```python
from build123d import *

# Parameters (mm, degrees)
F0_W           = 65
F0_H           = 38
F1_DEPTH       = 2
F2_W           = 34
F2_H           = 4
F3_DEPTH       = 48.95
F5_R           = 3.5
F6_DEPTH       = 3000
F4_R           = 25
F7_DEPTH       = 12
F9_R           = 3
F10_DEPTH      = 38
F11_R          = 25
F12_DEPTH      = 12
F12_DEPTH_BACK = 12


with BuildPart() as f1:
    # F0 (on Top) → F1 (new body)
    with BuildSketch(Plane.XY):
        Rectangle(F0_W, F0_H)
    extrude(amount=F1_DEPTH)

    # F2 (on face) → F3 (join)
    with BuildSketch(Plane(origin=(0, 0, 0), x_dir=(1, 0, 0), z_dir=(0, 0, -1))):
        with Locations((0, 17)):
            Rectangle(F2_W, F2_H)
        with Locations((0, -17)):
            Rectangle(F2_W, F2_H)
    extrude(amount=F3_DEPTH)

    # F5 (on face) → F6 (cut)
    with BuildSketch(Plane.XY.offset(2)):
        with Locations((27, 12)):
            Circle(F5_R)
        with Locations((27, -12)):
            Circle(F5_R)
        with Locations((-27, -12)):
            Circle(F5_R)
        with Locations((-27, 12)):
            Circle(F5_R)
    extrude(amount=-F6_DEPTH, mode=Mode.SUBTRACT)

    # F9 (on face) → F10 (join)
    with BuildSketch(Plane(origin=(0, 19, 0), x_dir=(-1, 0, 0), z_dir=(0, 1, 0))):
        with Locations((0, -43)):
            Circle(F9_R)
    extrude(amount=-F10_DEPTH)

    # F11 (on Front) → F12 (join, two sides)
    with BuildSketch(Plane.XZ) as f12_sk:
        with Locations((0, -43)):
            Circle(F11_R)
    extrude(amount=F12_DEPTH)
    extrude(f12_sk.sketch, amount=-F12_DEPTH_BACK)


with BuildPart() as f7:
    # F4 (on Front) → F7 (new body, symmetric)
    with BuildSketch(Plane.XZ):
        with Locations((0, -43)):
            Circle(F4_R)
    extrude(amount=F7_DEPTH, both=True)


solid = f1.part
```
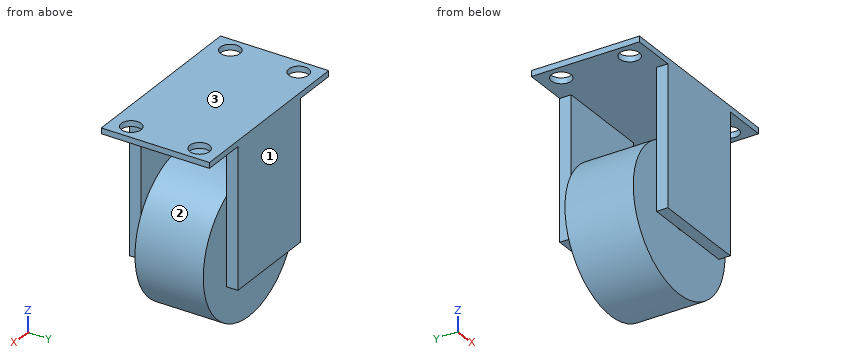
Can you work these out from the model? Positions are in its coordinate system, mm. Face numbers are marked on the shaded views. Round coordinates to 2 decimals unless told otherwise and drop trailing zeros. Loops run counter-clockwise (first coordinate to the right, second up) from the corner with the lowest first, then second, coordinate; pieces in that order, holes last. Notation, with made-up numbers: M 9.5,-29.75 L 51.5,-29.75 A19 ccw 51.5,4.25 Z; hole C 12.25,53 d4. An arc over 180 degrees is marked long. Answer as a JSON object with one key per item and string values. Group by question number.
Q1. Imagine slicing it at D-D, the plane z = -24.5. Please give me the cut outline in (x, y).
Q2. Imagine slicing it at B-B, the plane y = -1. Please give me the cut outline in (x, z), then the cut area to 3 significant figures.
Q3. Will these pins go through, and if not, where does the flat tip stop? pin 1 (3 mm diameter, centred on y = 7, z = -20, fed in from +X); pin 2 (10 mm diameter, centred on y = -8.5, z = -18, fed in from -X); pin 3 (10 mm diameter, centred on y = -2, z = -23.5, fed in from -X).
Q4. Imagine slicing it at A-A, the plane x = 27. Please give me the cut outline in (y, z), then the cut area to 3 significant figures.
Q5. Please list where these lines run through material, in increasing order: L1, parallel to Y at x = -27, z = 0.45; L2, parallel to Y at x = 16.5, z = -29; L3, parallel to Z at x = -4, y = -14.
Q6. We'd pull the mould along Z, two halves only. Please class the marked faces 1, 2 and 3: +Z half, -Z half, draft (parallel to the pull), parting line (faces both ways), or undercut.
Q7. Imagine slicing it at C-C, the plane x = 18. Please give me the cut outline in (y, z).
Findings:
{
 "1": {"outline": "M -17,-19 L 17,-19 L 17,-15 L -17,-15 Z; M -17,15 L 17,15 L 17,19 L -17,19 Z; M -16.82,-12 L 16.82,-12 L 16.82,12 L -16.82,12 Z"},
 "2": {"outline": "M -32.5,0 L 32.5,0 L 32.5,2 L -32.5,2 Z; C 0,-43 d50", "area": "2,090 mm2"},
 "3": {"pin 1": "stops at x = 12.76", "pin 2": "stops at x = -15", "pin 3": "stops at x = -20.37"},
 "4": {"outline": "M -19,0 L -15.5,0 L -15.5,2 L -19,2 Z; M -8.5,0 L 8.5,0 L 8.5,2 L -8.5,2 Z; M 15.5,0 L 19,0 L 19,2 L 15.5,2 Z", "area": "48.0 mm2"},
 "5": {"L1": "y = -19 to -15.5, -8.5 to 8.5, 15.5 to 19", "L2": "y = -19 to -15, -12 to 12, 15 to 19", "L3": "z = 0 to 2"},
 "6": {"face 1": "draft", "face 2": "undercut", "face 3": "+Z half"},
 "7": {"outline": "M -19,0 L 19,0 L 19,2 L -19,2 Z; M -12,-60.35 L 12,-60.35 L 12,-25.65 L -12,-25.65 Z"}
}
